Autodesk Inventor part; units mm, degrees
ref_plane "YZ Plane" through (0, 0, 0) normal (1, 0, 0) x (0, 1, 0)
ref_plane "XZ Plane" through (0, 0, 0) normal (0, 1, 0) x (-1, 0, 0)
ref_plane "XY Plane" through (0, 0, 0) normal (0, 0, 1) x (1, 0, 0)
sketch "Sketch1" plane through (0, 0, 0) normal (0, 1, 0) x (-1, 0, 0)
  line L0 (-21, -11.5) -> (-21, -16.5)
  line L1 (-21, -16.5) -> (0, -16.5)
  line L2 (0, -16.5) -> (0, 16.5) construction
  line L3 (0, 16.5) -> (-9, 16.5)
  line L4 (-9, 16.5) -> (-9, -11.5)
  line L5 (-9, -11.5) -> (-21, -11.5)
  line L6 (21, -11.5) -> (21, -16.5)
  line L7 (21, -16.5) -> (0, -16.5)
  line L8 (0, 16.5) -> (9, 16.5)
  line L9 (9, 16.5) -> (9, -11.5)
  line L10 (9, -11.5) -> (21, -11.5)
  point P0 (0, 0)
  point P1 (0, 0)
  dimension "d0" = 5
  dimension "d1" = 33
  dimension "d2" = 21
  dimension "d3" = 9
extrude "Extrusion1" add sketch "Sketch1" along normal mid plane 14
sketch "Sketch2" plane through (0, 7, 0) normal (0, 1, 0) x (1, 0, 0)
  arc A0 (0.75, -7.5054) -> (-0.75, -7.5054) centre (0, -3.5) ccw
  line L0 (-0.75, -16.5) -> (0.75, -16.5)
  line L1 (0.75, -16.5) -> (0.75, -7.5054)
  line L2 (-0.75, -7.5054) -> (-0.75, -16.5)
  line L3 (-9, -16.5) -> (9, -16.5)
  point P0 (0, 0)
  point P1 (0, -16.5)
  dimension "d6" = 8.15
  dimension "d7" = 13
  dimension "d8" = 1.5
extrude "Extrusion2" cut sketch "Sketch2" against normal through all
sketch "Sketch3" plane through (9, -7, -11.5) normal (1, 0, 0) x (0, 0, -1)
  circle A0 centre (-23.5, 7) radius 1.6
  line L0 (-28, 0) -> (-28, 14)
  point P0 (-11.5, 7)
  dimension "d11" = 3.2
  dimension "d13" = 4.5
extrude "Extrusion3" cut sketch "Sketch3" against normal through all
sketch "Sketch4" plane through (-9, -7, 16.5) normal (-1, 0, 0) x (0, 0, 1)
  circle A0 centre (-4.5, 7) radius 1.6
  line L0 (-6.1373, 4.15) -> (-2.8627, 4.15)
  line L1 (-2.8627, 4.15) -> (-1.25, 7)
  line L2 (-1.25, 7) -> (-2.8627, 9.85)
  line L3 (-2.8627, 9.85) -> (-6.1373, 9.85)
  line L4 (-6.1373, 9.85) -> (-7.75, 7)
  line L5 (-7.75, 7) -> (-6.1373, 4.15)
  point P0 (-16.5, 7)
  point P1 (-4.5, 4.15)
  point P2 (-4.5, 9.85)
  dimension "d16" = 5.7
  dimension "d17" = 6.5
extrude "Extrusion4" cut sketch "Sketch4" against normal blind 2.6
sketch "Sketch5" plane through (-21, 7, -11.5) normal (0, 0, 1) x (1, 0, 0)
  circle A0 centre (6, -7) radius 2.1
  circle A1 centre (36, -7) radius 2.1
  line L0 (0, -14) -> (0, 0)
  line L1 (0, 0) -> (12, 0)
  line L2 (30, 0) -> (42, 0)
  point P0 (21, -7)
  point P1 (0, -7)
  point P2 (6, 0)
  point P3 (36, 0)
  dimension "d20" = 4.2
extrude "Extrusion5" cut sketch "Sketch5" against normal through all
chamfer "Chamfer2" distance 1.5 angle 45 4 edges at (-21, 7, -14) (-21, -7, -14) (21, 7, -14) (21, -7, -14)
fillet "Fillet1" radius 1 2 edges at (-9, 0, 16.5) (9, 0, 16.5)
chamfer "Chamfer3" distance 1 angle 45 2 edges at (0, -7, -0.575) (0, 7, -0.575)
properties part number "SH8"
Source: CAD feature listing. Evaluate the final solid. Frame: model axes, mm. A direction names the side the tool comes from. Give positions to 0.01 mm unless a question says otherwise; leave off trailing zeros. Write each loop counter-clockwise with the first axis right and the second up, starting at its lowest first coordinate (ties: lowest second). Pieces come first, ordered by that corner, then holes. Notation, with made-up numbers: M -14,-21 L 26,-21 A21 cw 26,15 Z; hole C -35.75,65 d6. An arc over 180 degrees is marked long. Return JSON: item names as keys, results as strings. Group by question number.
1) Pin query (flat end, axial travel): P1, Ø5, axis at x = -15, y = 0, coming from the +Z side; P2, Ø1.7, axis at y = 0, z = 12.5, coming from the -X side; P3, Ø3, axis at y = 3.5, z = 7.5, coming from the -X side; P4, Ø7, axis at y = -2, z = 13.5, coming from the +X side. Return the tip coordinate at first contact, or that it passes through.
2) Material intervals for line 1 along Y through (x, z) = (7, 12); line 2 along Y through (x, z) = (-15, -14); line 3 along X through (y, z) = (1.5, -15), sorted ascending. Write a range as [from, to].
3) Pull-direction query (Z, two-part tool) for faces 1 (the face through (-4, 0, 16.5)), 2 (the face through (-17.1, 0.09, -13.96)), 3 (the face through (-7.718, 1.445, 9.568)); classes: pulls with the +Z half, pulls with the -Z half, needs draft (parallel to the pull), parting line crosses it, or undercut.
4) Cut plane D-D, the plane x = 7. Output: boundary loops of the cut face in (y, z), plus the area to 3 significant figures.
5) Cut plane C-C, the plane y = 3.75. Output: boundary loops of the cut face in (x, z), plus the area to 3 significant figures.
6) Set-up query: faces 4 (the face through (-7.718, -1.445, 14.432)), 5 (the face through (12, 0, -11.5)), 6 (the face through (-0.18, -6.17, -0.74)). Return all of +Z, -Z, +X, -X, +Y, -Y with unobstructed straight access to the full face (end or side cutting, diameter ignored); none if empty.
7) Cut plane A-A, the plane z = 12. Output: boundary loops of the cut face in (x, y).
8) Cut plane B-B, the plane x = 15. Output: boundary loops of the cut face in (y, z).
Recorded:
{
 "1": {"P1": "stops at z = -11.5", "P2": "passes through", "P3": "stops at x = -9", "P4": "stops at x = 9"},
 "2": {"line 1": "y = [-7, -1.6], [1.6, 7]", "line 2": "y = [-7, -2.1], [2.1, 7]", "line 3": "x = [-21, -16.47], [-13.53, 13.53], [16.47, 21]"},
 "3": {"face 1": "pulls with the +Z half", "face 2": "needs draft", "face 3": "undercut"},
 "4": {"outline": "M -7,-16.5 L 7,-16.5 L 7,16.5 L -7,16.5 Z; hole C 0,12 d3.2", "area": "454 mm²"},
 "5": {"outline": "M -21,-16.5 L 21,-16.5 L 21,-11.5 L 9,-11.5 L 9,15.5 A1 ccw 8,16.5 L 0.75,16.5 L 0.75,7.51 A4.08 cw long -0.75,7.51 L -0.75,16.5 L -8,16.5 A1 ccw -9,15.5 L -9,-11.5 L -21,-11.5 Z", "area": "648 mm²"},
 "6": {"face 4": "-X", "face 5": "+Z, +X, +Y, -Y", "face 6": "-Y"},
 "7": {"outline": "M -9,-7 L -0.75,-7 L -0.75,-1.6 L -6.4,-1.6 L -6.4,-2.85 L -9,-2.85 Z; M -9,2.85 L -6.4,2.85 L -6.4,1.6 L -0.75,1.6 L -0.75,7 L -9,7 Z; M 0.75,-7 L 9,-7 L 9,-1.6 L 0.75,-1.6 Z; M 0.75,1.6 L 9,1.6 L 9,7 L 0.75,7 Z"},
 "8": {"outline": "M -7,-16.5 L -2.1,-16.5 L -2.1,-11.5 L -7,-11.5 Z; M 2.1,-16.5 L 7,-16.5 L 7,-11.5 L 2.1,-11.5 Z"}
}
